from build123d import *

# Parameters (mm, degrees)
SKETCH_2_R         = 7.5
EXTRUDE_1_DEPTH    = 16
DOME_1_FACE_RADIUS = 7.5
DOME_1_HEIGHT      = 7
SKETCH_3_W         = 10
SKETCH_3_H         = 15
EXTRUDE_2_DEPTH    = 16
CHAMFER_1_SIZE     = 8
CHAMFER_1_SIZE2    = 3.730461265
HOLE_WIZARD_M4_1_D = 4.1


with BuildPart() as part:
    # 草图2 → 凸台-拉伸1 (new body)
    with BuildSketch(Plane.XY):
        Circle(SKETCH_2_R)
    extrude(amount=EXTRUDE_1_DEPTH)

    # 圆顶1: a dome of height H over a round flat face of radius A is a cap of a sphere of radius (A * A + H * H) / (2 * H)
    dome_1_r = (DOME_1_FACE_RADIUS * DOME_1_FACE_RADIUS + DOME_1_HEIGHT * DOME_1_HEIGHT) / (2 * DOME_1_HEIGHT)
    dome_1_base = Plane((0, 0, 16), z_dir=(0, 0, 1))
    with Locations(dome_1_base.offset(DOME_1_HEIGHT - dome_1_r)):
        dome_1_ball = Sphere(dome_1_r, mode=Mode.PRIVATE)
    add(split(dome_1_ball, bisect_by=dome_1_base, keep=Keep.TOP, mode=Mode.PRIVATE))

    # 草图3 → 凸台-拉伸2 (add)
    with BuildSketch(Plane(origin=(0, 0, 0), x_dir=(-1, 0, 0), z_dir=(0, 0, -1))):
        Rectangle(SKETCH_3_W, SKETCH_3_H)
    extrude(amount=EXTRUDE_2_DEPTH)

    # 倒角1
    chamfer_1_edges = [part.edges().sort_by_distance(p)[0] for p in [
        (0, -7.5, -16),
    ]]
    chamfer_1_side = [part.faces().sort_by_distance(p)[0] for p in [
        (0, -7.5, -8),
    ]]
    chamfer(chamfer_1_edges, length=CHAMFER_1_SIZE, length2=CHAMFER_1_SIZE2, reference=chamfer_1_side[0])

    # M4 间隙孔1 (through all)
    with Locations(Plane(origin=(5, 0, 0), x_dir=(0, 0, -1), z_dir=(1, 0, 0))):
        with Locations((7.921197697, 4.5), (11.302143791, -2.750462296)):
            Hole(HOLE_WIZARD_M4_1_D / 2)


solid = part.part
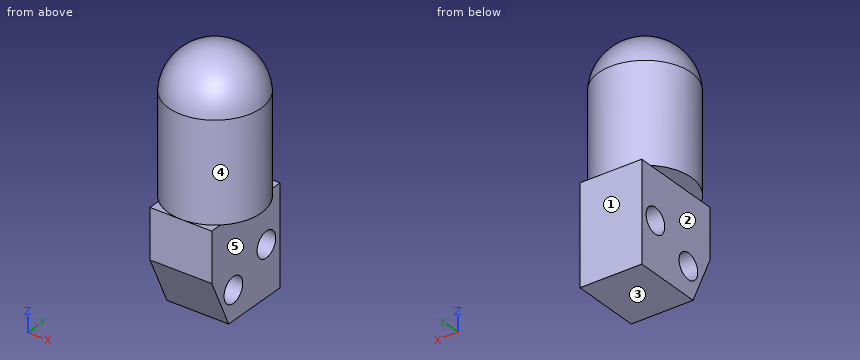
Can you work these out from the model? Positions are in its coordinate system, mm. Face numbers are marked on the shaded views. A direction names the side the tool comes from. Give positions to 0.01 mm unless a question says otherwise; leave off trailing zeros. Loops run counter-clockwise (first coordinate to the right, second up) from the corner with the lowest first, then second, coordinate; pieces in that order, holes last. Notation, with made-up numbers: (71.5, -19) -> (114.5, -19) arc R21 cw to (114.5, -2) -> close; hole circle Ø2 at (52.25, -20.75). An arc over 180 degrees is marked (long way). Return JSON: item names as keys, results as strings.
Q1. I need wall thicknesses on probe 1 along Z at (x, y) = (3.25, 3.5); probe 2 along Z at (x, y) = (3, -4.25); probe 3 along Y at (x, z) = (0.5, -12.5). Which ranges of each line are inside material? Lowest first, please.
Checks:
{"probe 1": "z = -16 to -9.71, -6.13 to 21.29", "probe 2": "z = -14.97 to -12.7, -9.9 to 20.91", "probe 3": "y = -5.4 to -4.41, -1.09 to 7.5"}
Q2. For pin 1 Ø4 at (x, y) = (-5.5, 1) entering from +Z; pin 2 Ø1 at (x, y) = (-2.5, 6.5) entering from +Z; pin 3 Ø2 at (x, y) = (3.5, 6.5) entering from +Z, each with a flat end and sliding along its axis, tell me the tip position at first contact or that it passes through.
Checks:
{"pin 1": "stops at z = 22.09", "pin 2": "stops at z = 19.32", "pin 3": "stops at z = 19.45"}
Q3. I want a section at A-A, the plane y = 4.5. List the corners of the cut face in (x, z) for me, then the cut area to 3 significant figures.
Checks:
{"outline": "(-6, 0) -> (-5, 0) -> (-5, -5.87) -> (5, -5.87) -> (5, 0) -> (6, 0) -> (6, 16) arc R6.02 ccw to (-6, 16) -> close; (-5, -16) -> (5, -16) -> (5, -9.97) -> (-5, -9.97) -> close", "area": "362 mm2"}
Q4. I want a section at B-B, the plane z = -7.5. List the corners of the cut face in (x, y) for me, then the cut area to 3 significant figures.
Checks:
{"outline": "(-5, -7.5) -> (5, -7.5) -> (5, 2.49) -> (-5, 2.49) -> close; (-5, 6.51) -> (5, 6.51) -> (5, 7.5) -> (-5, 7.5) -> close", "area": "110 mm2"}
Q5. I want a section at C-C, the plane x = -1.5. List the corners of the cut face in (y, z) for me, then the cut area to 3 significant figures.
Checks:
{"outline": "(-7.5, -8) -> (-3.77, -16) -> (7.5, -16) -> (7.5, 0) -> (7.35, 0) -> (7.35, 16) arc R7.37 ccw to (-7.35, 16) -> (-7.35, 0) -> (-7.5, 0) -> close; hole circle Ø4.1 at (-2.75, -11.3); hole circle Ø4.1 at (4.5, -7.92)", "area": "511 mm2"}
Q6. On a 3-axis mill with a long thin cutter (end or side, diameter ignored), from which of +Z, -Z, +X, -X, +Y, -Y can I reach the whole of each face in a straight line? I mean the marked faces 1, 2, 3, 4 and 5. Say none if no direction works.
Checks:
{"face 1": "+Z, -Z, +X, -X, +Y", "face 2": "-Z, -X, +Y, -Y", "face 3": "-Z, +X, -X, +Y, -Y", "face 4": "+Z", "face 5": "-Z, +X, +Y, -Y"}
Q7. I want a section at D-D, the plane y = 0. List the corners of the cut face in (x, z) for me, then the cut area to 3 significant figures.
Checks:
{"outline": "(-7.5, 0) -> (-5, 0) -> (-5, -16) -> (5, -16) -> (5, 0) -> (7.5, 0) -> (7.5, 16) arc R7.52 ccw to (-7.5, 16) -> close", "area": "481 mm2"}
